from build123d import *

# Parameters (mm, degrees)
F1_DEPTH = 25
F2_R     = 5


with BuildPart() as f1:
    # F0 (on Right) → F1 (new body)
    with BuildSketch(Plane.YZ):
        Polygon((0, -20), (0, 0), (-120, 0), (-120, -7), (-40, -20), align=None)
    extrude(amount=F1_DEPTH)

    # F2
    f2_edges = [f1.edges().sort_by_distance(p)[0] for p in [
        (25, -20, -20),
        (25, -80, -13.5),
        (12.5, -120, -7),
        (0, -80, -13.5),
        (0, -20, -20),
    ]]
    fillet(f2_edges, radius=F2_R)


solid = f1.part
Here's how the part is built. I have some questions about the finished solid (model axes, mm). Coordinates: 2 decimals unless noted, no trailing zeros. Write each loop counter-clockwise with the first axis right and the second up, starting at its lowest first coordinate (ties: lowest second). Pieces come first, ordered by that corner, then holes.
Item 1: If I drill on line 1 (Z direction, x = 10, y = -89); line 2 (Z direction, x = 8, y = -41.5); line 3 (X direction, y = -84.5, z = -8.25), over which ranges is the centre line in solid material (lowest first)?
Item 2: I want a section at A-A on x = 6. Write out the boundary of the cut face in (y, z).
Item 3: I want a section at B-B on y = -25. Write out the boundary of the cut face in (x, z).
Item 4: Will these pins go through, and if not, where does the flat tip stop? pin 1 (1 mm diameter, centred on x = 14, z = -4, fed in from -Y); pin 2 (6 mm diameter, centred on y = -50, z = -17, fed in from +X).
Findings below:
1. line 1: z = -12.04 to 0
1. line 2: z = -19.76 to 0
1. line 3: x = 0.03 to 24.97
2. outline: (-120, -2.75) arc R5 ccw to (-115.8, -7.68) - (-40, -20) - (0, -20) - (0, 0) - (-120, 0) - close
3. outline: (0, -15) arc R5 ccw to (5, -20) - (20, -20) arc R5 ccw to (25, -15) - (25, 0) - (0, 0) - close
4. pin 1: stops at y = -119.94
4. pin 2: stops at x = 24.96
